```python
from build123d import *

# Parameters (mm, degrees)
ESQUISSE2_W                = 308
ESQUISSE2_H                = 250
BOSS_EXTRU_1_DEPTH         = 1
ESQUISSE3_R                = 1.5
ENL_V_MAT_EXTRU_1_DEPTH    = 397.692576185
R_P_TITION_LIN_AIRE1_COUNT = 2
R_P_TITION_LIN_AIRE1_PITCH = 150
ESQUISSE4_R                = 15
ENL_V_MAT_EXTRU_2_DEPTH    = 397.692576185


with BuildPart() as part:
    # Esquisse2 → Boss.-Extru.1 (new body)
    with BuildSketch(Plane.XY):
        with Locations((154, 125)):
            Rectangle(ESQUISSE2_W, ESQUISSE2_H)
    extrude(amount=BOSS_EXTRU_1_DEPTH)

    # Esquisse3 → Enlèv. mat.-Extru.1 (cut, through all)
    with BuildSketch(Plane.XY.offset(1)):
        with Locations((10, 200)):
            Circle(ESQUISSE3_R)
        with Locations((298, 200)):
            Circle(ESQUISSE3_R)
    enl_v_mat_extru_1 = extrude(amount=-ENL_V_MAT_EXTRU_1_DEPTH, mode=Mode.SUBTRACT)

    # Répétition linéaire1: Enlèv. mat.-Extru.1 ×2
    with Locations(*[(0, -i * R_P_TITION_LIN_AIRE1_PITCH, 0) for i in range(1, R_P_TITION_LIN_AIRE1_COUNT)]):
        add(enl_v_mat_extru_1, mode=Mode.SUBTRACT)

    # Esquisse4 → Enlèv. mat.-Extru.2 (cut, through all)
    with BuildSketch(Plane.XY.offset(1)):
        with Locations((50, 200)):
            Circle(ESQUISSE4_R)
        with Locations((258, 200)):
            Circle(ESQUISSE4_R)
        with Locations((50, 50)):
            Circle(ESQUISSE4_R)
        with Locations((258, 50)):
            Circle(ESQUISSE4_R)
    extrude(amount=-ENL_V_MAT_EXTRU_2_DEPTH, mode=Mode.SUBTRACT)


solid = part.part
```
Geometry check sheet. Reference: the model listing, model coordinates, mm. Give positions to 0.01 mm unless a question says otherwise; leave off trailing zeros. Loops run counter-clockwise (first coordinate to the right, second up) from the corner with the lowest first, then second, coordinate; pieces in that order, holes last. Notation, with made-up numbers: M 21,-30.75 L 66,-30.75 A16 ccw 66,-22.75 Z; hole C 10.25,-5.5 d9. An arc over 180 degrees is marked long. Write item = value, one per line.
(1) Sectioned sample at B-B, the plane x = 258. Record the cut outline in (y, z), plus the area to 3 significant figures.
Answer below:
outline = M 0,0 L 35,0 L 35,1 L 0,1 Z; M 65,0 L 185,0 L 185,1 L 65,1 Z; M 215,0 L 250,0 L 250,1 L 215,1 Z
area = 190 mm2
(2) Release check for a two-part mould opening along Y. For faces 1 (the face through (152, 127, 0)), 2 (the face through (46.748, 185.357, 0.507)) record: released by +Y, released by -Y, zero draft, split by the parting line, or undercut.
Answer below:
face_1 = zero draft
face_2 = undercut
(3) Sectioned sample at A-A, the plane z = 0.8. State how many separate pieces and enclosed holes the cut face has, plus the area to 3 significant figures.
Answer below:
separate_pieces = 1
enclosed_holes = 8
area = 74,100 mm2
(4) Material ranges on line 1 (Y direction, x = 10, z = 0.3); line 2 (Y direction, x = 50, z = 0.5); line 3 (X direction, y = 50.5, z = 0.15), recorded low to high. Write a range as [from, to].
Answer below:
line_1 = [0, 48.5], [51.5, 198.5], [201.5, 250]
line_2 = [0, 35], [65, 185], [215, 250]
line_3 = [0, 8.59], [11.41, 35.01], [64.99, 243.01], [272.99, 296.59], [299.41, 308]
